Verification items for the finished model (mm, model axes). Face numbers are marked on the shaded views. Give positions to 0.01 mm unless a question says otherwise; leave off trailing zeros. Order: outer loops, then holes, each group sorted by start corner. A loop starts at its lowest first (then second) coordinate and runs counter-clockwise, first axis right, second up. Notation, with made-up numbers: (16, -33) - (60, -33) arc R29 ccw to (60, -2) - close; hole circle Ø4 at (27.25, 5.25). An arc over 180 degrees is marked (long way). Answer as a JSON object with one key per item and string values.
```python
from build123d import *

# Parameters (mm, degrees)
SKETCH1_R           = 400
BOSS_EXTRUDE1_DEPTH = 125
SKETCH2_R           = 37.5
BOSS_EXTRUDE2_DEPTH = 1500
SKETCH3_W           = 50
SKETCH3_H           = 500
BOSS_EXTRUDE3_DEPTH = 250
SKETCH4_R           = 18.75
SKETCH4_R_2         = 35
SKETCH4_W           = 125
SKETCH4_H           = 200
BOSS_EXTRUDE4_DEPTH = 75
FILLET1_R           = 62.5


with BuildPart() as part:
    # Sketch1 → Boss-Extrude1 (new body)
    with BuildSketch(Plane.XY):
        Circle(SKETCH1_R)
    extrude(amount=BOSS_EXTRUDE1_DEPTH)

    # Sketch2 → Boss-Extrude2 (add)
    with BuildSketch(Plane(origin=(0, 0, 0), x_dir=(-1, 0, 0), z_dir=(0, 0, -1))):
        with Locations(Location((0, 0, 0), (0, 0, 180))):
            Circle(SKETCH2_R)
    extrude(amount=BOSS_EXTRUDE2_DEPTH)

    # Sketch3 → Boss-Extrude3 (add)
    with BuildSketch(Plane(origin=(0, 0, -1500), x_dir=(-1, 0, 0), z_dir=(0, 0, -1))):
        with Locations((50, 210)):
            Rectangle(SKETCH3_W, SKETCH3_H)
    extrude(amount=BOSS_EXTRUDE3_DEPTH)

    # Sketch4 → Boss-Extrude4 (add)
    with BuildSketch(Plane.ZY.offset(25)):
        with Locations(Location((-1687.5, 60, 0), (0, 0, 270))):
            Circle(SKETCH4_R)
        with Locations(Location((-1625, 397.09, 0), (0, 0, 270))):
            Circle(SKETCH4_R_2)
        with Locations((-1562.5, 60)):
            Rectangle(SKETCH4_W, SKETCH4_H)
    extrude(amount=-BOSS_EXTRUDE4_DEPTH)

    # Fillet1
    # the kernel refuses this fillet: 62.5 mm, written as the material it takes off along each edge
    with BuildSketch(Plane(origin=(-231.25, 460, -1500), x_dir=(0, -1, 0), z_dir=(1, 0, 0))) as fillet1_piece_1:
        with BuildLine():
            CenterArc((FILLET1_R, FILLET1_R), FILLET1_R, 180, 90)
            Line((0, FILLET1_R), (0, 0))
            Line((0, 0), (FILLET1_R, 0))
        make_face()
    extrude(amount=362.5, mode=Mode.SUBTRACT)
    with BuildSketch(Plane(origin=(-231.25, -40, -1500), x_dir=(0, 1, 0), z_dir=(1, 0, 0))) as fillet1_piece_2_section:
        with BuildLine():
            CenterArc((FILLET1_R, -FILLET1_R), FILLET1_R, 90, 90)
            Line((0, -FILLET1_R), (0, 0))
            Line((0, 0), (FILLET1_R, 0))
        make_face()
    fillet1_piece_2 = extrude(amount=437.5, mode=Mode.PRIVATE)
    fillet1_piece_2 = fillet1_piece_2 - Plane(origin=(0, 0, -1501.420624631), x_dir=(1, 0, 0), z_dir=(0, 0, 1)) * Cylinder(37.5, 1125, mode=Mode.PRIVATE)
    add(fillet1_piece_2, mode=Mode.SUBTRACT)
    with BuildSketch(Plane(origin=(-231.25, 460, -1750), x_dir=(0, -1, 0), z_dir=(1, 0, 0)), Plane(origin=(131.25, -40, -1750), x_dir=(0, 1, 0), z_dir=(-1, 0, 0))) as fillet1_piece_3:
        with BuildLine():
            CenterArc((FILLET1_R, -FILLET1_R), FILLET1_R, 90, 90)
            Line((0, -FILLET1_R), (0, 0))
            Line((0, 0), (FILLET1_R, 0))
        make_face()
    extrude(amount=362.5, mode=Mode.SUBTRACT)


solid = part.part
```
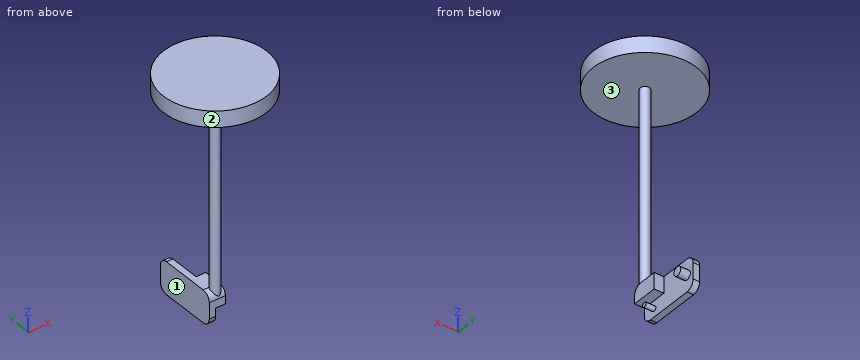
(1) Material ranges on line 1 along X through (y, z) = (3.5, -391.5); line 2 along Z through (x, y) = (-221.5, 95); line 3 along Z through (x, y) = (5, 159.5), recorded low to high. Write a range as [from, to].
Computed values:
{"line 1": "x = [-37.34, 37.34]", "line 2": "z = [0, 125]", "line 3": "z = [-1625, -1500], [0, 125]"}
(2) Section check D-D (z = -855.5). Record the cut outline in (x, y), then the cut area to 3 significant figures.
Computed values:
{"outline": "circle Ø75 at (0, 0)", "area": "4,420 mm²"}
(3) Release check for a two-part mould opening along X. For the marked faces 1, 2 and 3 record: pulls with the +X half, pulls with the -X half, needs draft (parallel to the pull), parting line crosses it, or undercut.
Computed values:
{"face 1": "pulls with the -X half", "face 2": "parting line crosses it", "face 3": "needs draft"}
(4) Section check C-C (y = 0). Record the cut outline in (x, z), then the cut area to 3 significant figures.
Computed values:
{"outline": "(-400, 0) - (-37.5, 0) - (-37.5, -1504.19) - (-75, -1504.19) - (-75, -1745.81) - (-25, -1745.81) - (-25, -1625) - (50, -1625) - (50, -1504.19) - (37.5, -1504.19) - (37.5, 0) - (400, 0) - (400, 125) - (-400, 125) - close", "area": "234,000 mm²"}
(5) Section check B-B (y = 186.5). Record the cut outline in (x, z).
Computed values:
{"outline": "(-353.86, 0) - (353.86, 0) - (353.86, 125) - (-353.86, 125) - close; (-75, -1750) - (-25, -1750) - (-25, -1500) - (-75, -1500) - close"}
(6) Gauge pin test, flat ends, axial feed: pin 1 Ø10 at (x, y) = (-242, 230.5) entering from -Z; pin 2 Ø19 at (y, z) = (63.5, -1686.5) entering from +X. Record the tip position at first contact, or that the pin passes through.
Computed values:
{"pin 1": "stops at z = 0", "pin 2": "stops at x = 50"}
(7) Section check A-A (x = 0). Record the cut outline in (y, z).
Computed values:
{"outline": "(-400, 0) - (-37.5, 0) - (-37.5, -1545) arc R62.5 ccw to (-40, -1562.5) - (-40, -1625) - (160, -1625) - (160, -1500) - (37.5, -1500) - (37.5, 0) - (400, 0) - (400, 125) - (-400, 125) - close; circle Ø37.5 at (60, -1687.5); circle Ø70 at (397.09, -1625)"}
